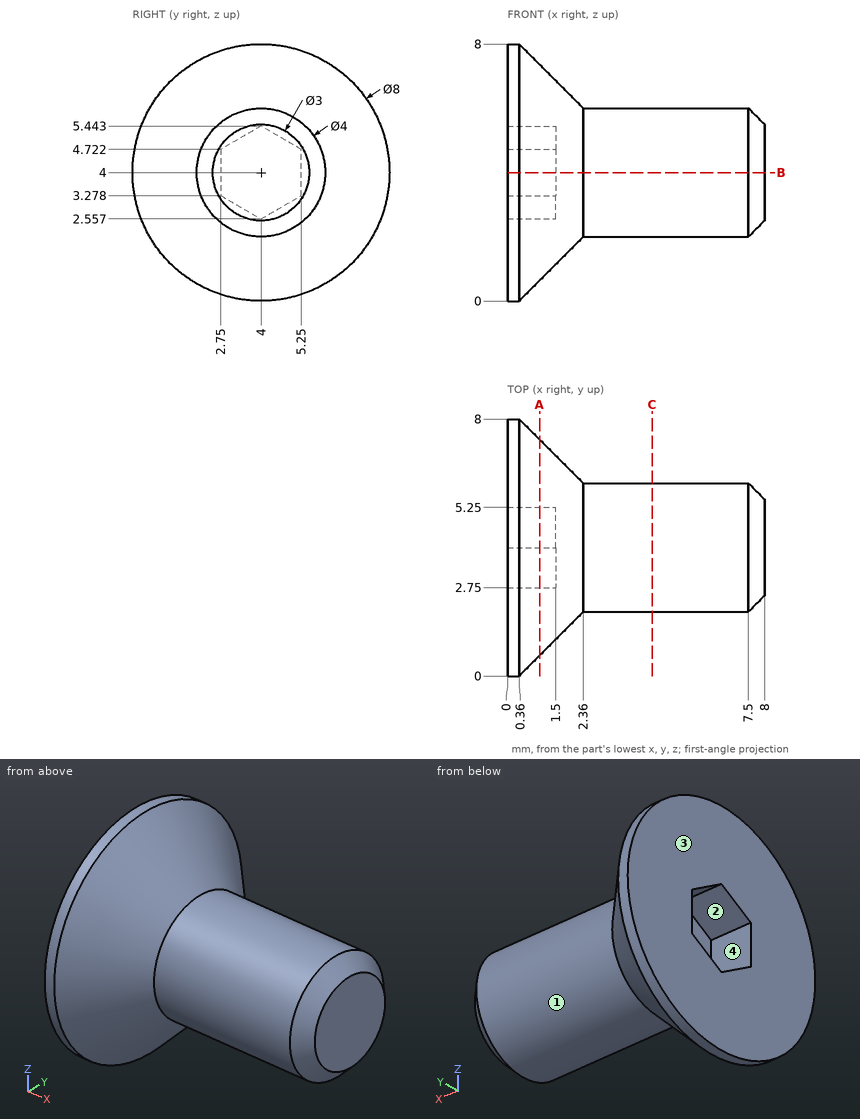
Drawing for the job (mm, zero at the part's lowest x, y, z). Round coordinates to 2 decimals unless told otherwise and drop trailing zeros. Loops run counter-clockwise (first coordinate to the right, second up) from the corner with the lowest first, then second, coordinate; pieces in that order, holes last. Notation, with made-up numbers: (-6, 33.5) -> (-1, 33.5) arc R21 ccw to (-1, 55.5) -> close; hole circle Ø10 at (-36.75, 34.5). An arc over 180 degrees is marked (long way). Use one line per item in the form item = value. Start each with the question number.
Item 1: Band-saw the part on B-B (z = 4). List the corners of the cut face in (x, y).
Item 2: Drop a flat-ended pin along its axis: pin 1 Ø1 at (x, z) = (1.5, 4) entering from -Y. Give the stop position or say it passes through.
Item 3: Drill centre lines: line 1 along X through (y, z) = (4.75, 4.25); line 2 along Z through (x, y) = (0.5, 3.5) (1 decimal); line 3 along Y through (x, z) = (4, 4.5). Where is each one in solid material? Low to high.
Item 4: Band-saw the part on A-A (x = 1). List the corners of the cut face in (y, z).
Item 5: Band-saw the part on C-C (x = 4.5). List the corners of the cut face in (y, z), plus the area to 3 significant figures.
Item 6: Two-plate mould, pull along Z, no slides. Class the marked faces 1, 2, 3 and 4: released by +Z, released by -Z, zero draft, split by the parting line, or undercut.
Data:
q1.outline = (0, 0) -> (0.36, 0) -> (2.36, 2) -> (7.5, 2) -> (8, 2.5) -> (8, 5.5) -> (7.5, 6) -> (2.36, 6) -> (0.36, 8) -> (0, 8) -> (0, 5.25) -> (1.5, 5.25) -> (1.5, 2.75) -> (0, 2.75) -> close
q2.pin_1 = 0.64
q3.line_1 = 1.5 to 8
q3.line_2 = 0.2 to 2.8, 5.2 to 7.8
q3.line_3 = 2.06 to 5.94
q4.outline = circle Ø6.72 at (4, 4); hole (2.75, 3.28) -> (4, 2.56) -> (5.25, 3.28) -> (5.25, 4.72) -> (4, 5.44) -> (2.75, 4.72) -> close
q5.outline = circle Ø4 at (4, 4)
q5.area = 12.6 mm^2
q6.face_1 = split by the parting line
q6.face_2 = undercut
q6.face_3 = zero draft
q6.face_4 = undercut
